For this review, take the finished solid that the model builds, in its own axes (mm). A direction names the side the tool comes from. Give positions to 0.01 mm unless a question says otherwise; leave off trailing zeros. Write each loop counter-clockwise with the first axis right and the second up, starting at its lowest first coordinate (ties: lowest second). Pieces come first, ordered by that corner, then holes.
from build123d import *

# Parameters (mm, degrees)
SKETCH1_W           = 13.2
SKETCH1_H           = 20.6
BOSS_EXTRUDE1_DEPTH = 15.5
SKETCH2_R           = 1.5
BOSS_EXTRUDE2_DEPTH = 4
SKETCH3_W           = 13.2
SKETCH3_H           = 3.8
BOSS_EXTRUDE3_DEPTH = 0.5
CUT_EXTRUDE1_DEPTH  = 11
SKETCH5_W           = 4.1
SKETCH5_H           = 2.2
CUT_EXTRUDE2_DEPTH  = 5
SKETCH6_W           = 13.5
SKETCH6_H           = 1.2
BOSS_EXTRUDE5_DEPTH = 1
SKETCH7_W           = 13.5
SKETCH7_H           = 1.2
BOSS_EXTRUDE6_DEPTH = 1
SKETCH8_W           = 13.2
SKETCH8_H           = 8.722289783
CUT_EXTRUDE3_DEPTH  = 0.5


with BuildPart() as part:
    # Sketch1 → Boss-Extrude1 (new body)
    with BuildSketch(Plane.XY):
        Rectangle(SKETCH1_W, SKETCH1_H)
    extrude(amount=BOSS_EXTRUDE1_DEPTH)

    # Sketch2 → Boss-Extrude2 (add)
    with BuildSketch(Plane(origin=(0, 0, 0), x_dir=(-1, 0, 0), z_dir=(0, 0, -1))):
        with Locations((5.08, 0)):
            Circle(SKETCH2_R)
        with Locations((-5.08, 0)):
            Circle(SKETCH2_R)
    extrude(amount=BOSS_EXTRUDE2_DEPTH)

    # Sketch3 → Boss-Extrude3 (add)
    with BuildSketch(Plane.XY.offset(15.5)):
        with Locations((0, -8.4)):
            Rectangle(SKETCH3_W, SKETCH3_H)
    extrude(amount=BOSS_EXTRUDE3_DEPTH)

    # Sketch4 → Cut-Extrude1 (cut)
    with BuildSketch(Plane.XZ.offset(10.3)):
        Polygon((-3.6, 15), (3.6, 15), (3.6, 13), (4.6, 13), (4.6, 11), (5.6, 11), (5.6, 8.4), (4.6, 8.4), (4.6, 6.1), (3.6, 6.1), (3.6, 4), (-3.6, 4), (-3.6, 6.1), (-4.6, 6.1), (-4.6, 8.4), (-5.6, 8.4), (-5.6, 11), (-4.6, 11), (-4.6, 13), (-3.6, 13), align=None)
    extrude(amount=-CUT_EXTRUDE1_DEPTH, mode=Mode.SUBTRACT)

    # Sketch5 → Cut-Extrude2 (cut)
    with BuildSketch(Plane.XZ.offset(10.3)):
        with Locations((0.05, 2.9)):
            Rectangle(SKETCH5_W, SKETCH5_H)
    extrude(amount=-CUT_EXTRUDE2_DEPTH, mode=Mode.SUBTRACT)

    # Sketch6 → Boss-Extrude5 (add)
    with BuildSketch(Plane.ZY.offset(6.6)):
        with Locations((7.75, -7.4)):
            Rectangle(SKETCH6_W, SKETCH6_H)
    extrude(amount=BOSS_EXTRUDE5_DEPTH)

    # Sketch7 → Boss-Extrude6 (add)
    with BuildSketch(Plane(origin=(6.6, 0, 0), x_dir=(0, 0, -1), z_dir=(1, 0, 0))):
        with Locations((-7.75, -6.2)):
            Rectangle(SKETCH7_W, SKETCH7_H)
    extrude(amount=BOSS_EXTRUDE6_DEPTH)

    # Sketch8 → Cut-Extrude3 (cut)
    with BuildSketch(Plane(origin=(0, 0, 0), x_dir=(-1, 0, 0), z_dir=(0, 0, -1))):
        with Locations((0, -5.938855109)):
            Rectangle(SKETCH8_W, SKETCH8_H)
    extrude(amount=-CUT_EXTRUDE3_DEPTH, mode=Mode.SUBTRACT)


solid = part.part
(1) For L1, parallel to X at y = -1.75, z = 5.75; L2, parallel to Z at x = 0.25, y = -6.75; L3, parallel to Z at x = 2.75, y = -6.75, list the stretches that pass through material, from the lowest coordinate up.
(2) We need section D-D (x = 0). Write out the cut boundary in (y, z).
(3) Clearance check with flat-ended pins moving along their axes: pin 1 Ø1.1 at (x, y) = (5, -7) entering from -Z; pin 2 Ø5 at (x, z) = (1, 12) entering from -Y; pin 3 Ø2 at (y, z) = (-5, 13.5) entering from -X. State where each tip first meets the part, or that it passes through.
(4) The part is to be moulded in two halves that separate along X. For faces 1 (the flat face through (-7.6, -7, 8)), 2 (the flat face through (5, -5, 8.4)), 3 (the flat face through (5, 0, -4)), say which applies: +X half, -X half, draft (parallel to the pull), parting line (faces both ways), or undercut.
(5) We need section B-B (x = -5.08). Write out the cut boundary in (y, z).
(6) We need section C-C (z = 13.5). Write out the cut boundary in (x, y), and give its area (3 significant figures).
(7) Tool access review of faces 4 (the flat face through (-7, -6.8, 8)), 5 (the flat face through (0, -6, 0.5)), 6 (the flat face through (7, -6.8, 8)), 7 (the flat face through (4, -5, 13)): name each direction out of +Z, -Z, +X, -X, +Y, -Y from which nothing blocks a thin tool from reaching the whole face with its end or side.
The answers:
1. L1: x = -6.6 to -3.6, 3.6 to 6.6
1. L2: z = 0.5 to 1.8, 15 to 16
1. L3: z = 0.5 to 4, 15 to 16
2. outline: (-10.3, 0.5) - (-1.58, 0.5) - (-1.58, 0) - (10.3, 0) - (10.3, 15.5) - (-6.5, 15.5) - (-6.5, 16) - (-10.3, 16) - (-10.3, 15) - (0.7, 15) - (0.7, 4) - (-5.3, 4) - (-5.3, 1.8) - (-10.3, 1.8) - close
3. pin 1: stops at z = 0.5
3. pin 2: stops at y = 0.7
3. pin 3: stops at x = -6.6
4. face 1: -X half
4. face 2: undercut
4. face 3: draft
5. outline: (-10.3, 0.5) - (-1.58, 0.5) - (-1.58, 0) - (-1.5, 0) - (-1.5, -4) - (1.5, -4) - (1.5, 0) - (10.3, 0) - (10.3, 15.5) - (-6.5, 15.5) - (-6.5, 16) - (-10.3, 16) - (-10.3, 11) - (0.7, 11) - (0.7, 8.4) - (-10.3, 8.4) - close
6. outline: (-7.6, -8) - (-6.6, -8) - (-6.6, -10.3) - (-3.6, -10.3) - (-3.6, 0.7) - (3.6, 0.7) - (3.6, -10.3) - (6.6, -10.3) - (6.6, -6.8) - (7.6, -6.8) - (7.6, -5.6) - (6.6, -5.6) - (6.6, 10.3) - (-6.6, 10.3) - (-6.6, -6.8) - (-7.6, -6.8) - close
6. area: 195 mm2
7. face 4: +Z, -Z, -X, +Y
7. face 5: -Z, +X, -X, -Y
7. face 6: +Z, -Z, +X, -Y
7. face 7: -Y
